from build123d import *

# Parameters (mm, degrees)
EXTRUDE_1_DEPTH          = 25
FILLET_2_R               = 15
CUT_EXTRUDE_2_DEPTH      = 121.632707028
CUT_EXTRUDE_2_DEPTH_BACK = 121.632707028
SKETCH_9_R               = 2.5
CUT_EXTRUDE_3_DEPTH      = 120.533468117
PATTERN_LINEAR_1_COUNT   = 2
PATTERN_LINEAR_1_PITCH   = 24
CUT_EXTRUDE_4_DEPTH      = 14
SKETCH_11_R              = 7.5
SKETCH_11_R_2            = 3.25
EXTRUDE_3_DEPTH          = 14
PATTERN_LINEAR_2_COUNT   = 2
PATTERN_LINEAR_2_PITCH   = 195


with BuildPart() as part:
    # Эскиз4 → Бобышка-Вытянуть1 (new body)
    with BuildSketch(Plane(origin=(0, 0, 0), x_dir=(0, 0, -1), z_dir=(1, 0, 0))):
        with BuildLine():
            Line((-25, 26.5), (25, 26.5))
            Line((25, 26.5), (99.487179761, 17.5))
            ThreePointArc((99.487179761, 17.5), (115, 0), (99.487179761, -17.5))
            Line((99.487179761, -17.5), (25, -26.5))
            Line((25, -26.5), (-25, -26.5))
            Line((-25, -26.5), (-99.487179761, -17.5))
            ThreePointArc((-99.487179761, -17.5), (-115, 0), (-99.487179761, 17.5))
            Line((-99.487179761, 17.5), (-25, 26.5))
        make_face()
    extrude(amount=EXTRUDE_1_DEPTH)

    # Скругление2
    # the kernel refuses this fillet: 15 mm, written as the material it takes off along each edge
    with BuildSketch(Plane(origin=(25, 30.998265024, 12.229230609), x_dir=(-1, 0, 0), z_dir=(0, -0.11995373398361225, -0.9927794829182304)), Plane(origin=(25, 17.5, 99.487179761), x_dir=(-1, 0, 0), z_dir=(0, 0.11995373398361225, -0.9927794829182304)), Plane(origin=(25, -30.998265024, -12.229230609), x_dir=(-1, 0, 0), z_dir=(0, 0.11995373398361238, 0.9927794829182304)), Plane(origin=(25, -17.5, -99.487179761), x_dir=(-1, 0, 0), z_dir=(0, -0.1199537339836124, 0.9927794829182304))) as fillet_2_piece_1:
        with BuildLine():
            CenterArc((FILLET_2_R, -FILLET_2_R), FILLET_2_R, 90, 90)
            Line((0, -FILLET_2_R), (0, 0))
            Line((0, 0), (FILLET_2_R, 0))
        make_face()
    extrude(amount=112.528927413, mode=Mode.SUBTRACT)
    with BuildSketch(Plane(origin=(25, 0, -97.372721938), x_dir=(0, 0.9927794829182303, -0.11995373398361334), z_dir=(0, 0.11995373398361334, 0.9927794829182303))) as fillet_2_piece_2:
        with BuildLine():
            CenterArc((17.627278062 - FILLET_2_R, FILLET_2_R), FILLET_2_R, 270, 90)
            Line((17.627278062 - FILLET_2_R, 0), (17.627278062, 0))
            Line((17.627278062, 0), (17.627278062, FILLET_2_R))
        make_face()
    revolve(axis=Axis((25, 0, -97.372721938), (-1, 0, 0)), revolution_arc=166.221135111, mode=Mode.SUBTRACT)
    with BuildSketch(Plane(origin=(25, 0, 97.372721938), x_dir=(0, -0.9927794829182303, 0.11995373398361334), z_dir=(0, -0.11995373398361334, -0.9927794829182303))) as fillet_2_piece_3:
        with BuildLine():
            CenterArc((17.627278062 - FILLET_2_R, FILLET_2_R), FILLET_2_R, 270, 90)
            Line((17.627278062 - FILLET_2_R, 0), (17.627278062, 0))
            Line((17.627278062, 0), (17.627278062, FILLET_2_R))
        make_face()
    revolve(axis=Axis((25, 0, 97.372721938), (-1, 0, 0)), revolution_arc=166.221135111, mode=Mode.SUBTRACT)

    # Эскиз8 → Вырез-Вытянуть2 (cut, two sides: drawn at the far end of the back side and taken through both)
    with BuildSketch(Plane(origin=(0, 0, 0), x_dir=(1, 0, 0), z_dir=(0, 1, 0)).offset(-CUT_EXTRUDE_2_DEPTH_BACK)):
        Polygon((19, -27.152763866), (19, 24.847236134), (28, 31.474618083), (28, -33.525381917), align=None)
    extrude(amount=CUT_EXTRUDE_2_DEPTH + CUT_EXTRUDE_2_DEPTH_BACK, mode=Mode.SUBTRACT)

    # Эскиз9 → Вырез-Вытянуть3 (cut, through all)
    with BuildSketch(Plane(origin=(19, 0, 0), x_dir=(0, 0, -1), z_dir=(1, 0, 0))):
        with Locations((-16.652763866, 8)):
            Circle(SKETCH_9_R)
        with Locations((-16.652763866, -8)):
            Circle(SKETCH_9_R)
    cut_extrude_3 = extrude(amount=-CUT_EXTRUDE_3_DEPTH, mode=Mode.SUBTRACT)

    # Линейный массив1: Вырез-Вытянуть3 ×2
    with Locations(*[(0, 0, -i * PATTERN_LINEAR_1_PITCH) for i in range(1, PATTERN_LINEAR_1_COUNT)]):
        add(cut_extrude_3, mode=Mode.SUBTRACT)

    # Эскиз10 → Вырез-Вытянуть4 (cut)
    with BuildSketch(Plane.ZY):
        with BuildLine():
            Line((99.007364825, 13.528882068), (24.759223266, 22.5))
            Line((24.759223266, 22.5), (-24.759223266, 22.5))
            Line((-24.759223266, 22.5), (-99.007364825, 13.528882068))
            ThreePointArc((-99.007364825, 13.528882068), (-111, 0), (-99.007364825, -13.528882068))
            Line((-99.007364825, -13.528882068), (-24.759223266, -22.5))
            Line((-24.759223266, -22.5), (24.759223266, -22.5))
            Line((24.759223266, -22.5), (99.007364825, -13.528882068))
            ThreePointArc((99.007364825, -13.528882068), (111, 0), (99.007364825, 13.528882068))
        make_face()
    extrude(amount=-CUT_EXTRUDE_4_DEPTH, mode=Mode.SUBTRACT)

    # Эскиз11 → Бобышка-Вытянуть3 (add)
    with BuildSketch(Plane.ZY.offset(-14)):
        with Locations((97.552941864, 0)):
            Circle(SKETCH_11_R)
        with Locations((97.552941864, 0)):
            Circle(SKETCH_11_R_2, mode=Mode.SUBTRACT)
    extrude_3 = extrude(amount=EXTRUDE_3_DEPTH)

    # Линейный массив2: Бобышка-Вытянуть3 ×2
    with Locations(*[(0, 0, -i * PATTERN_LINEAR_2_PITCH) for i in range(1, PATTERN_LINEAR_2_COUNT)]):
        add(extrude_3)


solid = part.part
Source: CAD feature listing. Evaluate the final solid. Frame: model axes, mm. A direction names the side the tool comes from. Coordinates: 2 decimals unless noted, no trailing zeros. Loops run counter-clockwise (first coordinate to the right, second up) from the corner with the lowest first, then second, coordinate; pieces in that order, holes last. Notation, with made-up numbers: (22.5, -39.5) - (45.5, -39.5) arc R31 ccw to (45.5, -0.5) - close; hole circle Ø11 at (72.25, 9). An arc over 180 degrees is marked (long way). Return JSON: item names as keys, results as strings.
Q1. Material intervals for line 1 along Y through (x, z) = (11.5, -9); line 2 along Z through (x, y) = (10.75, 1.5); line 3 along Z through (x, y) = (14.75, -6), sorted ascending.
Results:
{"line 1": "-26.5 to -22.5, 22.5 to 26.5", "line 2": "-114.92 to -110.92, -104.8 to -100.33, -94.56 to -90.1, 90.2 to 94.67, 100.44 to 104.9, 110.92 to 114.92", "line 3": "-113.12 to -8.85, -5.85 to 15.15, 18.15 to 113.12"}
Q2. Section A-A, the plane x = 7.75. Return loops of the section in (y, z), plus the area to 3 significant figures.
Results:
{"outline": "(-26.5, -25) - (-17.5, -99.49) arc R17.63 ccw to (17.5, -99.49) - (26.5, -25) - (26.5, 25) - (17.5, 99.49) arc R17.63 ccw to (-17.5, 99.49) - (-26.5, 25) - close; circle Ø15 at (0, -97.45); circle Ø15 at (0, 97.55); hole (-22.5, -24.76) - (-13.53, -99.01) arc R13.63 ccw to (13.53, -99.01) - (22.5, -24.76) - (22.5, 24.76) - (13.53, 99.01) arc R13.63 ccw to (-13.53, 99.01) - (-22.5, 24.76) - close; hole circle Ø6.5 at (0, -97.45); hole circle Ø6.5 at (0, 97.55)", "area": "2,250 mm2"}
Q3. Contact query for flat-ended pins moving along their axis: P1, Ø8, axis at x = 20, z = -62, coming from the -Y side; P2, Ø1.5, axis at y = -9.5, z = -55, coming from the -X side; P3, Ø4, axis at x = 6.5, y = -7.5, coming from the +Z side. Output: stop coordinate, or through.
Results:
{"P1": "y = -20.83", "P2": "x = 14", "P3": "z = 114.12"}
Q4. Mould query, pull axis Z, two halves, no side actions, for faces 4 (the cylindrical face through (20.489, 17.827, 61.118)), 5 (the flat face through (4.93, 22.063, -61.722)), 6 (the cylindrical face through (7, 0, 111)). Classes: released by +Z, released by -Z, zero draft, split by the parting line, or undercut.
Results:
{"face 4": "released by +Z", "face 5": "released by -Z", "face 6": "undercut"}
Q5. Access query for faces 1 (the flat face through (7, 22.5, 0)), 2 (the flat face through (25, 0, -57)), 3 (the flat face through (21.958, -0.329, -27.025)). Directions: +Z, -Z, +X, -X, +Y, -Y. A direction counts if a zero-diameter tool reaches every point of the face in a straight line with its end or side. Return the directions, or none.
Results:
{"face 1": "-X", "face 2": "+Z, -Z, +X, +Y, -Y", "face 3": "+X, +Y, -Y"}
